Check sheet for the modelled part. Datum: model origin and axes. Units: mm. Face numbers are marked on the shaded views. Round coordinates to 2 decimals unless told otherwise and drop trailing zeros. Loops run counter-clockwise (first coordinate to the right, second up) from the corner with the lowest first, then second, coordinate; pieces in that order, holes last. Notation, with made-up numbers: (25, -24) - (76, -24) arc R15 cw to (76, -5) - close; hole circle Ø6 at (-22, -39). An arc over 180 degrees is marked (long way). Put each result on its own line as item: value.
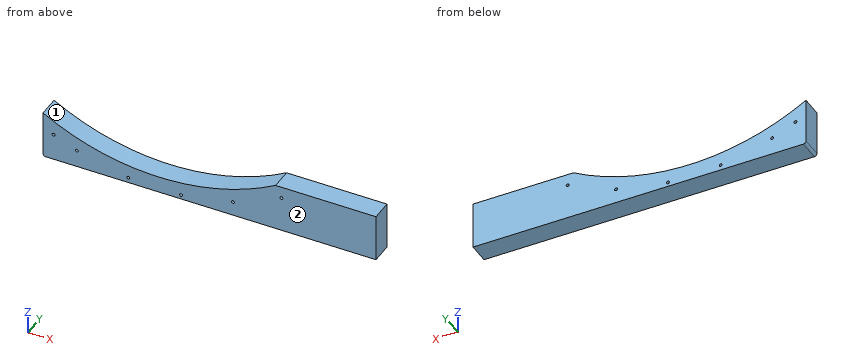
Autodesk Inventor part; units mm, degrees
ref_plane "YZ Plane" through (0, 0, 0) normal (1, 0, 0) x (0, 1, 0)
ref_plane "XZ Plane" through (0, 0, 0) normal (0, 1, 0) x (-1, 0, 0)
ref_plane "XY Plane" through (0, 0, 0) normal (0, 0, 1) x (1, 0, 0)
sketch "Sketch1" plane through (0, 0, 0) normal (0, 1, 0) x (-1, 0, 0)
  line L0 (0, 329.241) -> (0, -329.241) construction
  line L1 (203.5937, 0) -> (-203.5937, 0) construction
  arc A0 (-441.1, 0) -> (220, -382.3208) centre (0, 0) ccw
  line L2 (-441.1, 0) -> (-441.1, 400)
  line L3 (-441.1, 400) -> (-500, 400)
  line L4 (-500, 400) -> (-500, -500)
  line L5 (-500, -500) -> (220, -500)
  line L6 (220, -500) -> (220, -382.3208)
  dimension "d0" = 500
  dimension "d1" = 400
  dimension "d2" = 500
  dimension "d3" = 441.1
  dimension "d4" = 720
extrude "Extrusion1" add sketch "Sketch1" along normal blind 40
sketch "Sketch3" plane through (0, 0, 0) normal (0, -1, 0) x (1, 0, 0)
  line L0 (-480, -472.3208) -> (410, -472.3208)
  line L1 (410, -472.3208) -> (410, -382.3208)
  line L2 (410, -382.3208) -> (-480, -382.3208)
  line L3 (-480, -382.3208) -> (-480, -472.3208)
  arc A0 (-220, -382.3208) -> (441.1, 0) centre (0, 0) ccw
  line L4 (500, 400) -> (500, -500)
  line L5 (-944.7434, 629.3425) -> (927.6453, 629.3425)
  line L6 (927.6453, 629.3425) -> (927.6453, -768.0218)
  line L7 (927.6453, -768.0218) -> (-944.7434, -768.0218)
  line L8 (-944.7434, -768.0218) -> (-944.7434, 629.3425)
  dimension "d44" = 890
  dimension "d45" = 90
  dimension "d71" = 90
sketch "Sketch4" plane through (0, 0, 0) normal (0, -1, 0) x (1, 0, 0)
  line L0 (441.1, 400) -> (500, 400) construction
  line L1 (441.1, 0) -> (441.1, 400) construction
  arc A0 (-220, -382.3208) -> (441.1, 0) centre (0, 0) ccw construction
  line L2 (464.3817, -39.9852) -> (0, 0) construction
  line L3 (0, 0) -> (445.1648, -138.1214) construction
  line L4 (423.7332, -194.1633) -> (0, 0) construction
  line L5 (360.2723, -295.7246) -> (0, 0) construction
  line L6 (289.0138, -365.6778) -> (0, 0) construction
  line L7 (389.8771, -255.4312) -> (0, 0) construction
  line L8 (326.5218, -332.615) -> (0, 0) construction
  line L9 (230.9911, -404.8361) -> (0, 0) construction
  line L10 (139.32, -444.7911) -> (0, 0) construction
  line L11 (41.2359, -464.2723) -> (0, 0) construction
  line L12 (464.3817, -39.9852) -> (445.1648, -138.1214) construction
  line L13 (445.1648, -138.1214) -> (423.7332, -194.1633) construction
  line L14 (423.7332, -194.1633) -> (389.8771, -255.4312) construction
  line L15 (389.8771, -255.4312) -> (360.2723, -295.7246) construction
  line L16 (360.2723, -295.7246) -> (326.5218, -332.615) construction
  line L17 (326.5218, -332.615) -> (289.0138, -365.6778) construction
  line L18 (289.0138, -365.6778) -> (230.9911, -404.8361) construction
  line L19 (230.9911, -404.8361) -> (139.32, -444.7911) construction
  line L20 (139.32, -444.7911) -> (41.2359, -464.2723) construction
  line L21 (-58.7462, -462.3831) -> (0, 0) construction
  line L22 (-156.0243, -439.2102) -> (0, 0) construction
  line L23 (-200, -421.0098) -> (0, 0) construction
  line L24 (41.2359, -464.2723) -> (-58.7462, -462.3831) construction
  line L25 (-58.7462, -462.3831) -> (-156.0243, -439.2102) construction
  line L26 (-200, -421.0098) -> (-156.0243, -439.2102) construction
  line L27 (-220, -500) -> (-220, -382.3208) construction
  point P0 (466.1, 360)
  point P1 (466.1, 260)
  point P2 (466.1, 160)
  point P3 (466.1, 60)
  dimension "d50" = 40
  dimension "d51" = 100
  dimension "d52" = 100
  dimension "d53" = 100
  dimension "d54" = 25
  dimension "d55" = 466.1
  dimension "d56" = 100
  dimension "d57" = 100
  dimension "d58" = 60
  dimension "d59" = 70
  dimension "d60" = 50
  dimension "d61" = 70
  dimension "d62" = 100
  dimension "d63" = 20
hole "Hole1" at (-200, 0, -421.0098) at (-156.0243, 0, -439.2102) at (-58.7462, 0, -462.3831) at (41.2359, 0, -464.2723) at (139.32, 0, -444.7911) at (230.9911, 0, -404.8361) at (289.0138, 0, -365.6778) at (326.5218, 0, -332.615) at (360.2723, 0, -295.7246) at (389.8771, 0, -255.4312) at (423.7332, 0, -194.1633) at (445.1648, 0, -138.1214) at (464.3817, 0, -39.9852) at (466.1, 0, 60) at (466.1, 0, 160) at (466.1, 0, 260) at (466.1, 0, 360) direction (0, 1, 0) diameter 5.5 end through all
extrude "Extrusion2" cut sketch "Sketch3" against normal through all
fillet "Fillet1" radius 5 1 edges at (-220, 20, -472.3208)
properties part number "boundaryV1"
Item 1: Section check C-C on x = -96. Enter the section's corners in (y, z), then the cut area to 3 significant figures.
Filled sheet:
outline: (0, -472.32) - (40, -472.32) - (40, -430.53) - (0, -430.53) - close
area: 1,670 mm²
Item 2: Section check B-B on x = 167.5. Enter the section's corners in (y, z), then the cut area to 3 significant figures.
Filled sheet:
outline: (0, -472.32) - (40, -472.32) - (40, -408.06) - (0, -408.06) - close
area: 2,570 mm²
Item 3: Release check for a two-part mould opening along X. For the marked faces 1 and 2 record: +X half, -X half, draft (parallel to the pull), parting line (faces both ways), or undercut.
Filled sheet:
face 1: undercut
face 2: draft
Item 4: Section check A-A on y = 29. Enter the section's corners in (x, z).
Filled sheet:
outline: (-220, -467.32) arc R5 ccw to (-215, -472.32) - (410, -472.32) - (410, -382.32) - (220, -382.32) arc R441.1 cw to (-220, -382.32) - close; hole circle Ø5.5 at (-200, -421.01); hole circle Ø5.5 at (-156.02, -439.21); hole circle Ø5.5 at (-58.75, -462.38); hole circle Ø5.5 at (41.24, -464.27); hole circle Ø5.5 at (139.32, -444.79); hole circle Ø5.5 at (230.99, -404.84)
Item 5: Thickness scan on line 1 (X direction, y = 14.5, z = -445); line 2 (X direction, y = 15.5, z = -406); line 3 (Z direction, x = 139.32, y = 13). Record the ranges inside material, lowest first. Write a range as from..to.
Filled sheet:
line 1: -220..136.58, 142.06..410
line 2: -220..-172.43, 172.43..228.5, 233.48..410
line 3: -472.32..-447.54, -442.04..-418.52
Item 6: Go/stop test with a flat-tipped pin: pin 1 (6.5 mm diameter, centred on x = 139.32, z = -444.79, fed in from +Y). Record where the tip stops, or that it passes through.
Filled sheet:
pin 1: y = 40
